```python
from build123d import *

# Parameters (mm, degrees)
CROQUIS1_W              = 28
CROQUIS1_H              = 28
CROQUIS1_R              = 8.05
SALIENTE_EXTRUIR1_DEPTH = 0.5
CROQUIS2_W              = 28
CROQUIS2_H              = 28
CROQUIS2_R              = 8.6
SALIENTE_EXTRUIR2_DEPTH = 6
CORTAR_EXTRUIR1_DEPTH   = 3.5
CROQUIS6_R              = 1.5
CORTAR_EXTRUIR2_DEPTH   = 23.5
CROQUIS7_W              = 2.5
CROQUIS7_H              = 5
CROQUIS7_W_2            = 10
CROQUIS7_H_2            = 3.5
SALIENTE_EXTRUIR3_DEPTH = 3
REDONDEO1_R             = 5


with BuildPart() as part:
    # Croquis1 → Saliente-Extruir1 (new, symmetric)
    with BuildSketch(Plane.XY):
        Rectangle(CROQUIS1_W, CROQUIS1_H)
        Circle(CROQUIS1_R, mode=Mode.SUBTRACT)
    extrude(amount=SALIENTE_EXTRUIR1_DEPTH, both=True)

    # Croquis2 → Saliente-Extruir2 (add)
    with BuildSketch(Plane.XY.offset(0.5)):
        Rectangle(CROQUIS2_W, CROQUIS2_H)
        Circle(CROQUIS2_R, mode=Mode.SUBTRACT)
    extrude(amount=SALIENTE_EXTRUIR2_DEPTH)

    # Croquis3 → Cortar-Extruir1 (cut)
    with BuildSketch(Plane.XY.offset(6.5)):
        Polygon((11.029978213, 12.15), (7.970021787, 12.15), (6.440043573, 9.5), (7.970021787, 6.85), (11.029978213, 6.85), (12.559956427, 9.5), align=None)
        Polygon((-6.440043573, 9.5), (-7.970021787, 12.15), (-11.029978213, 12.15), (-12.559956427, 9.5), (-11.029978213, 6.85), (-7.970021787, 6.85), align=None)
        Polygon((-7.970021787, -6.85), (-11.029978213, -6.85), (-12.559956427, -9.5), (-11.029978213, -12.15), (-7.970021787, -12.15), (-6.440043573, -9.5), align=None)
        Polygon((11.029978213, -6.85), (7.970021787, -6.85), (6.440043573, -9.5), (7.970021787, -12.15), (11.029978213, -12.15), (12.559956427, -9.5), align=None)
    extrude(amount=-CORTAR_EXTRUIR1_DEPTH, mode=Mode.SUBTRACT)

    # Croquis6 → Cortar-Extruir2 (cut)
    with BuildSketch(Plane(origin=(0, 0, -0.5), x_dir=(-1, 0, 0), z_dir=(0, 0, -1))):
        with Locations((-9.5, 9.5)):
            Circle(CROQUIS6_R)
        with Locations((9.5, 9.5)):
            Circle(CROQUIS6_R)
        with Locations((9.5, -9.5)):
            Circle(CROQUIS6_R)
        with Locations((-9.5, -9.5)):
            Circle(CROQUIS6_R)
    extrude(amount=-CORTAR_EXTRUIR2_DEPTH, mode=Mode.SUBTRACT)

    # Croquis7 → Saliente-Extruir3 (add)
    with BuildSketch(Plane(origin=(0, 0, -0.5), x_dir=(-1, 0, 0), z_dir=(0, 0, -1))):
        with Locations((-15.25, 0)):
            Rectangle(CROQUIS7_W, CROQUIS7_H)
        with Locations((0, -15.75)):
            Rectangle(CROQUIS7_W_2, CROQUIS7_H_2)
        Polygon((14, -2.5), (14, -5), (18.9, -5), (18.9, -2.5), (16.5, -2.5), align=None)
        with Locations((15.25, 0)):
            Rectangle(CROQUIS7_W, CROQUIS7_H)
        Polygon((14, 5), (14, 2.5), (16.5, 2.5), (18.9, 2.5), (18.9, 5), align=None)
    extrude(amount=-SALIENTE_EXTRUIR3_DEPTH)

    # Redondeo1
    redondeo1_edges = [part.edges().sort_by_distance(p)[0] for p in [
        (14, -14, 3),
        (-14, -14, 3),
        (-14, 14, 3),
        (14, 14, 3),
    ]]
    fillet(redondeo1_edges, radius=REDONDEO1_R)


solid = part.part
```
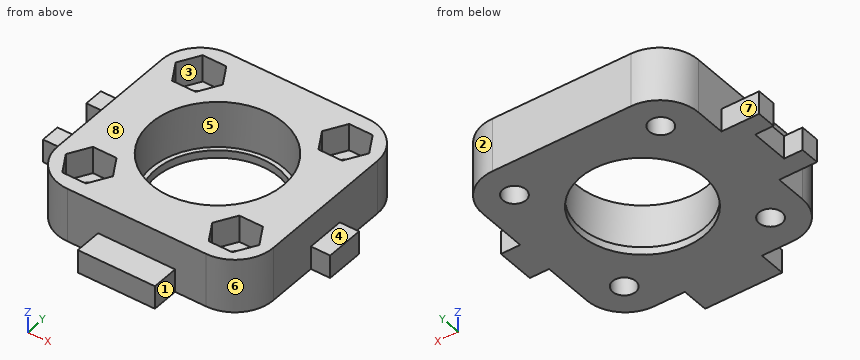
Check sheet for the modelled part. Datum: model origin and axes. Units: mm. Face numbers are marked on the shaded views. A direction names the side the tool comes from. Coordinates: 2 decimals unless noted, no trailing zeros. Order: outer loops, then holes, each group sorted by start corner. A loop starts at its lowest first (then second) coordinate and runs counter-clockwise, first axis right, second up. Notation, with made-up numbers: M -29,-15.5 L 30,-15.5 A18 ccw 30,-9.5 Z; hole C -24.5,17.25 d9. An arc over 180 degrees is marked long. Write each question's results on one line, items separated by ' | '. Start each with the question number.
1. Go/stop test with flat-tipped pins: P1, Ø0.8, axis at x = 15.5, z = 1.5, coming from the +Y side; P2, Ø0.9, axis at x = -9.5, z = 5, coming from the -Y side; P3, Ø4, axis at x = 9.5, y = -9.5, coming from the +Z side. Record where each tip stops, or that it passes through.
2. Material ranges on probe 1 along Y at (x, z) = (-9.5, 2.1); probe 2 along X at (y, z) = (-11, 5.5); probe 3 along Z at (x, y) = (10, -7.5), recorded low to high.
3. Cross-section at B-B on z = 4. State how many separate pieces and enclosed holes the cut face has, and give its area (3 significant figures).
4. Cross-section at A-A on y = 0. Record the cut outline in (x, z), and give its area (3 significant figures).
5. Access from +Z, -Z, +X, -X, +Y, -Y to the whole of each face (thin tool, end or side, straight path). Record for the marked faces 1, 2, 3 and 4.
6. Mould release check, pull along Y, two halves, no side actions. Record for the marked faces 5, 6, 7 and 8: +Y half, -Y half, draft (parallel to the pull), parting line (faces both ways), or undercut.
7. Cross-section at C-C on x = 2. Record the cut outline in (y, z).
Checks:
1) P1: stops at y = 2.5 | P2: stops at y = -14 | P3: stops at z = 3
2) probe 1: y = -13.97 to -11, -8 to 8, 11 to 13.97 | probe 2: x = -13.58 to -11.69, -7.31 to 7.31, 11.69 to 13.58 | probe 3: z = -0.5 to 3
3) separate pieces: 1 | enclosed holes: 5 | area: 433 mm²
4) outline: M -16.5,-0.5 L -8.05,-0.5 L -8.05,0.5 L -8.6,0.5 L -8.6,6.5 L -14,6.5 L -14,2.5 L -16.5,2.5 Z; M 8.05,-0.5 L 16.5,-0.5 L 16.5,2.5 L 14,2.5 L 14,6.5 L 8.6,6.5 L 8.6,0.5 L 8.05,0.5 Z | area: 91.7 mm²
5) face 1: +Z, -Z, +X, -Y | face 2: +Z, -Z, +X, +Y | face 3: +Z | face 4: +Z, +X, +Y, -Y
6) face 5: undercut | face 6: -Y half | face 7: +Y half | face 8: draft
7) outline: M -17.5,-0.5 L -7.8,-0.5 L -7.8,0.5 L -8.36,0.5 L -8.36,6.5 L -14,6.5 L -14,2.5 L -17.5,2.5 Z; M 7.8,-0.5 L 14,-0.5 L 14,6.5 L 8.36,6.5 L 8.36,0.5 L 7.8,0.5 Z
